Here's how the part is built. I have some questions about the finished solid (model axes, mm). A direction names the side the tool comes from. Coordinates: 2 decimals unless noted, no trailing zeros. Write each loop counter-clockwise with the first axis right and the second up, starting at its lowest first coordinate (ties: lowest second). Pieces come first, ordered by that corner, then holes. Notation, with made-up numbers: (-1.75, 23) -> (40.25, 23) arc R20 cw to (40.25, 55) -> close; hole circle Ø10 at (19.5, 78.25). An arc over 180 degrees is marked (long way). Use a Markdown table: item, result. Add a question column.
Item 1: Imagine slicing it at A-A, the plane z = 23. Write out the boundary of the cut face in (x, y).
Item 2: If I drill on line 1 along Y through (x, z) = (-15.5, 19); line 2 along X through (y, z) = (15, 30), over which ranges is the centre line in solid material (lowest first)? Write a range as from..to.
Item 3: Will these pins go through, and if not, where does the flat tip stop? pin 1 Ø4 at (x, y) = (11.5, 10.5) entering from -Z; pin 2 Ø2 at (x, y) = (-15.5, -15.5) entering from +Z (1 decimal); pin 3 Ø10 at (y, z) = (-4, 48.5) entering from +X; pin 4 Ø10 at (x, y) = (16.5, -17) entering from +Z.
Item 4: On a 3-axis mill with a long thin cutter (end or side, diameter ignored), from which of +Z, -Z, +X, -X, +Y, -Y can I reach the whole of each face in a straight line? I mean faces 1 (the cylindrical face through (-0.867, -3.905, 55.956)), 2 (the flat face through (0, -21.15, 21)). Say none if no direction works.
Item 5: Imagine slicing it at C-C, the plane y = -9. Write out the boundary of the cut face in (x, z).
Item 6: Imagine slicing it at D-D, the plane z = 60.5. Write out the boundary of the cut face in (x, y).
Item 7: Imagine slicing it at B-B, the plane x = 0. Write out the boundary of the cut face in (y, z).
```python
from build123d import *

# Parameters (mm, degrees)
F0_W     = 42.3
F0_H     = 42.3
F0_R     = 4
F1_DEPTH = 42.3
F2_DEPTH = 70


with BuildPart() as f1:
    # F0 (on Top) → F1 (new body)
    with BuildSketch(Plane.XY):
        Rectangle(F0_W, F0_H)
        with BuildLine():
            ThreePointArc((-15.5, 13.8), (-16.702082, 16.702082), (-13.8, 15.5))
            Line((-13.8, 15.5), (13.8, 15.5))
            ThreePointArc((13.8, 15.5), (15.5, 17.2), (17.2, 15.5))
            ThreePointArc((17.2, 15.5), (16.702082, 14.297918), (15.5, 13.8))
            Line((15.5, 13.8), (15.5, -13.8))
            ThreePointArc((15.5, -13.8), (16.702082, -14.297918), (17.2, -15.5))
            ThreePointArc((17.2, -15.5), (15.5, -17.2), (13.8, -15.5))
            Line((13.8, -15.5), (-13.8, -15.5))
            ThreePointArc((-13.8, -15.5), (-16.702082, -16.702082), (-15.5, -13.8))
            Line((-15.5, -13.8), (-15.5, 13.8))
        make_face(mode=Mode.SUBTRACT)
        with BuildLine():
            Line((13.8, 15.5), (-13.8, 15.5))
            ThreePointArc((-13.8, 15.5), (-14.297918, 14.297918), (-15.5, 13.8))
            Line((-15.5, 13.8), (-15.5, -13.8))
            ThreePointArc((-15.5, -13.8), (-14.297918, -14.297918), (-13.8, -15.5))
            Line((-13.8, -15.5), (13.8, -15.5))
            ThreePointArc((13.8, -15.5), (14.297918, -14.297918), (15.5, -13.8))
            Line((15.5, -13.8), (15.5, 13.8))
            ThreePointArc((15.5, 13.8), (14.297918, 14.297918), (13.8, 15.5))
        make_face()
        Circle(F0_R, mode=Mode.SUBTRACT)
        Circle(F0_R)
    extrude(amount=F1_DEPTH)

    # F0 (on Top) → F2 (join)
    with BuildSketch(Plane.XY):
        Circle(F0_R)
    extrude(amount=F2_DEPTH)


solid = f1.part
```
Ans:
| question | item | result |
|---|---|---|
| 1 | outline | (-21.15, -21.15) -> (21.15, -21.15) -> (21.15, 21.15) -> (-21.15, 21.15) -> close; hole (-15.5, -13.8) arc R1.7 ccw (long way) to (-13.8, -15.5) arc R1.7 ccw to start; hole (-15.5, 13.8) arc R1.7 ccw to (-13.8, 15.5) arc R1.7 ccw (long way) to start; hole (13.8, -15.5) arc R1.7 ccw to (17.2, -15.5) arc R1.7 ccw to (15.5, -13.8) arc R1.7 ccw to start; hole (13.8, 15.5) arc R1.7 ccw to (15.5, 13.8) arc R1.7 ccw to (17.2, 15.5) arc R1.7 ccw to start |
| 2 | line 1 | y = -21.15..-17.2, -13.8..13.8, 17.2..21.15 |
| 2 | line 2 | x = -21.15..-17.12, -13.88..13.88, 17.12..21.15 |
| 3 | pin 1 | stops at z = 0 |
| 3 | pin 2 | passes through |
| 3 | pin 3 | stops at x = 4 |
| 3 | pin 4 | stops at z = 42.3 |
| 4 | face 1 | +Z |
| 4 | face 2 | +Z, -Z, +X, -X, -Y |
| 5 | outline | (-21.15, 0) -> (21.15, 0) -> (21.15, 42.3) -> (-21.15, 42.3) -> close |
| 6 | outline | circle Ø8 at (0, 0) |
| 7 | outline | (-21.15, 0) -> (21.15, 0) -> (21.15, 42.3) -> (4, 42.3) -> (4, 70) -> (-4, 70) -> (-4, 42.3) -> (-21.15, 42.3) -> close |
